Geometry check sheet. Reference: drawing and pictorial views, mm from the part's lowest x, y, z. Give positions to 0.01 mm unless a question says otherwise; leave off trailing zeros. Write each loop counter-clockwise with the first axis right and the second up, starting at its lowest first coordinate (ties: lowest second). Pieces come first, ordered by that corner, then holes. Notation, with made-up numbers: (-36.75, 3.5) -> (12.25, 3.5) arc R25 cw to (12.25, 22.5) -> close; hole circle Ø6 at (-29.5, 32.5). An arc over 180 degrees is marked (long way). Answer as CSV lines item,"result".
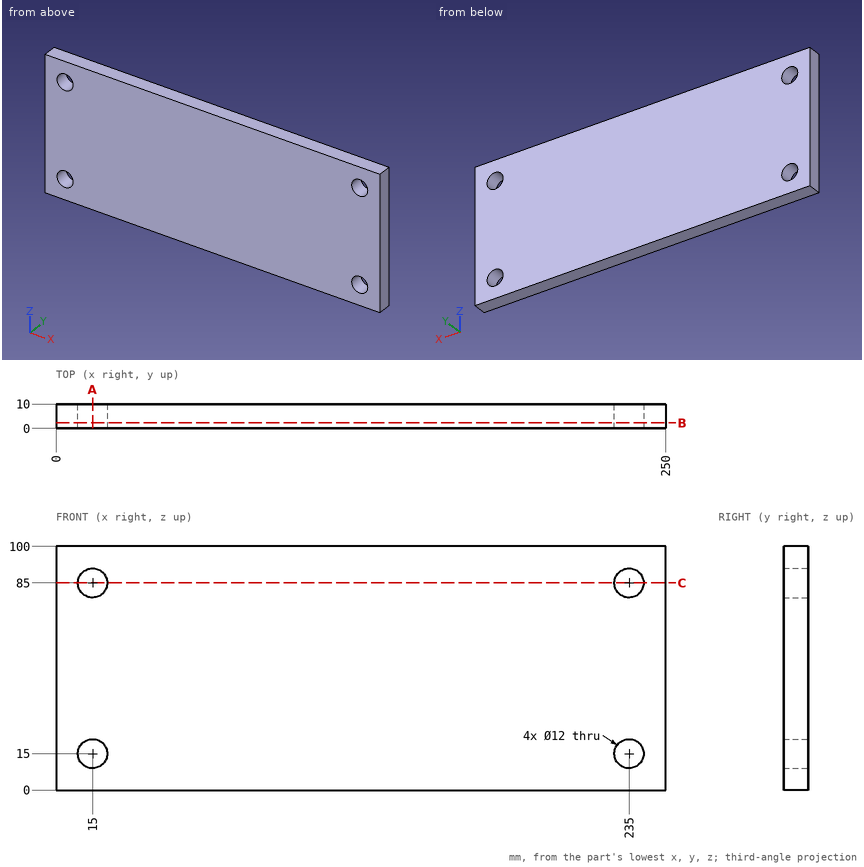
1) Section check A-A (x = 15). Record the boundary of the cut face in (y, z), and give its area (3 significant figures).
Reported:
outline,"(0, 0) -> (10, 0) -> (10, 9) -> (0, 9) -> close; (0, 21) -> (10, 21) -> (10, 79) -> (0, 79) -> close; (0, 91) -> (10, 91) -> (10, 100) -> (0, 100) -> close"
area,"760 mm²"
2) Scan lines: line 1 along Z through (x, y) = (235, 8); line 2 along X through (y, z) = (8, 85); line 3 along Z through (x, y) = (18.5, 5.5). Record each from-to range of solid material in increasing order.
Reported:
line 1,"0 to 9, 21 to 79, 91 to 100"
line 2,"0 to 9, 21 to 229, 241 to 250"
line 3,"0 to 10.13, 19.87 to 80.13, 89.87 to 100"
3) Depth check by flat-ended pin: pin 1 (11 mm diameter, centred on x = 235, z = 85, fed in from +Y); pin 2 (6 mm diameter, centred on x = 132, z = 25, fed in from -Y). Enter the tip coordinate at first touch or a pass-through.
Reported:
pin 1,"through"
pin 2,"y = 0"
4) Section check C-C (z = 85). Record the boundary of the cut face in (x, y).
Reported:
outline,"(0, 0) -> (9, 0) -> (9, 10) -> (0, 10) -> close; (21, 0) -> (229, 0) -> (229, 10) -> (21, 10) -> close; (241, 0) -> (250, 0) -> (250, 10) -> (241, 10) -> close"
5) Section check B-B (y = 2.25). Record the boundary of the cut face in (x, z).
Reported:
outline,"(0, 0) -> (250, 0) -> (250, 100) -> (0, 100) -> close; hole circle Ø12 at (15, 15); hole circle Ø12 at (15, 85); hole circle Ø12 at (235, 15); hole circle Ø12 at (235, 85)"
